from build123d import *

# Parameters (mm, degrees)
F0_W     = 203.2
F0_H     = 101.6
F1_DEPTH = 101.6
F2_W     = 76.2
F2_H     = 101.6
F3_DEPTH = 50.8
F4_W     = 127
F4_H     = 50.8
F5_DEPTH = 25.4


with BuildPart() as f1:
    # F0 (on Front) → F1 (new body)
    with BuildSketch(Plane.XZ):
        with Locations((4.342319, 12.05778)):
            Rectangle(F0_W, F0_H)
    extrude(amount=F1_DEPTH)

    # F2 (on face) → F3 (cut)
    with BuildSketch(Plane.XY.offset(62.85778)):
        with Locations((67.842319, -50.8)):
            Rectangle(F2_W, F2_H)
    extrude(amount=-F3_DEPTH, mode=Mode.SUBTRACT)

    # F4 (on face) → F5 (cut)
    with BuildSketch(Plane.XY.offset(62.85778)):
        with Locations((-33.757681, -50.8)):
            Rectangle(F4_W, F4_H)
    extrude(amount=-F5_DEPTH, mode=Mode.SUBTRACT)


solid = f1.part
Here's how the part is built. I have some questions about the finished solid (model axes, mm). A direction names the side the tool comes from. Give positions to 0.01 mm unless a question says otherwise; leave off trailing zeros. Order: outer loops, then holes, each group sorted by start corner. A loop starts at its lowest first (then second) coordinate and runs counter-clockwise, first axis right, second up. Notation, with made-up numbers: (68.5, 2.25) -> (105.5, 2.25) arc R31 cw to (105.5, 35.25) -> close; hole circle Ø9 at (13.5, 57.25). An arc over 180 degrees is marked (long way). Use a Markdown table: item, result. Add a question column.
Item 1: I need wall thicknesses on line 1 (Y direction, x = 29, z = 57); line 2 (Z direction, x = 27, y = -64); line 3 (X direction, y = -11, z = 55). Which ranges of each line are inside material? Lowest first, please.
Item 2: If we mould it in two halves opening along Y, with no side actions, what happens to faces 1 (the face through (105.942, -50, -14)), 2 (the face through (-35, -25.4, 50)), 3 (the face through (-20, 0, 13))? For each: pulls with the +Y half, pulls with the -Y half, needs draft (parallel to the pull), parting line crosses it, or undercut.
Item 3: Will these pins go through, and if not, where does the flat tip stop? pin 1 (10 mm diameter, centred on x = -11, y = -62, fed in from +Z); pin 2 (15 mm diameter, centred on y = -68, z = 43, fed in from +X).
Item 4: Imagine slicing it at D-D on y = -91.5. Please give me the cut outline in (x, z).
Item 5: Imagine slicing it at C-C on z = 33.5. Please give me the cut outline in (x, y), plus the area to 3 significant figures.
Item 6: Imagine slicing it at B-B on y = -64.5. Please give me the cut outline in (x, z).
Item 7: Imagine slicing it at A-A on x = -37.5. Please give me the cut outline in (y, z), plus the area to 3 significant figures.
Item 8: For faces 4 (the face through (-35, -76.2, 50)), 5 (the face through (29.742, -52, 32)), 6 (the face through (-35, -13, 62.858)), which set-ups out of +Z, -Z, +X, -X, +Y, -Y let a thin tool reach every point of the face, with its end or its side?
Data:
| question | item | result |
|---|---|---|
| 1 | line 1 | y = -101.6 to -76.2, -25.4 to 0 |
| 1 | line 2 | z = -38.74 to 37.46 |
| 1 | line 3 | x = -97.26 to 29.74 |
| 2 | face 1 | needs draft |
| 2 | face 2 | undercut |
| 2 | face 3 | pulls with the +Y half |
| 3 | pin 1 | stops at z = 37.46 |
| 3 | pin 2 | stops at x = 29.74 |
| 4 | outline | (-97.26, -38.74) -> (105.94, -38.74) -> (105.94, 12.06) -> (29.74, 12.06) -> (29.74, 62.86) -> (-97.26, 62.86) -> close |
| 5 | outline | (-97.26, -101.6) -> (29.74, -101.6) -> (29.74, 0) -> (-97.26, 0) -> close |
| 5 | area | 12,900 mm² |
| 6 | outline | (-97.26, -38.74) -> (105.94, -38.74) -> (105.94, 12.06) -> (29.74, 12.06) -> (29.74, 37.46) -> (-97.26, 37.46) -> close |
| 7 | outline | (-101.6, -38.74) -> (0, -38.74) -> (0, 62.86) -> (-25.4, 62.86) -> (-25.4, 37.46) -> (-76.2, 37.46) -> (-76.2, 62.86) -> (-101.6, 62.86) -> close |
| 7 | area | 9,030 mm² |
| 8 | face 4 | +Z, +X, -X |
| 8 | face 5 | +Z, +X, +Y, -Y |
| 8 | face 6 | +Z, +X, -X, +Y, -Y |
